```python
from build123d import *
from build123d.topology import SkipClean

# Parameters (mm, degrees)
SWEEP1_PROFILE_R = 12.5


with BuildPart() as part:
    # Sweep1: sweep along a path in Sketch1
    with BuildLine(Plane.XY) as sweep1_path:
        Line((120, -20), (20, -20))
        ThreePointArc((20, -20), (5.857864376, -14.142135624), (0, 0))
        Line((0, 0), (0, 314.65))
        ThreePointArc((0, 314.65), (-8.037977367, 341.838024139), (-29.567546263, 360.28457937))
        Line((-29.567546263, 360.28457937), (-73.011665824, 379.736275328))
    # Sweep1 profile (on start of the path) → Sweep1 (sweep)
    with BuildSketch(Plane(origin=(120, -20, 0), x_dir=(0, 0, -1), z_dir=(-1, 0, 0))):
        Circle(SWEEP1_PROFILE_R)
    sweep(path=sweep1_path.line)

    # Sketch16 → Revolve1 (revolve)
    with SkipClean():  # the faces are left unmerged after this step: merging them gives an invalid solid
        with BuildSketch(Plane.XY):
            with BuildLine():
                Line((120, -7.5), (120, -32.5))
                ThreePointArc((120, -32.5), (132.5, -20), (120, -7.5))
            make_face()
        revolve(axis=Axis((120, -7.5, 0), (0, -1, 0)))


solid = part.part
```
Source: CAD feature listing. Evaluate the final solid. Frame: model axes, mm. Coordinates: 2 decimals unless noted, no trailing zeros. Order: outer loops, then holes, each group sorted by start corner. A loop starts at its lowest first (then second) coordinate and runs counter-clockwise, first axis right, second up. Notation, with made-up numbers: M 35.5,52.5 L 50.5,52.5 A22 ccw 50.5,86.5 Z; hole C 4.25,46 d1. An arc over 180 degrees is marked long. Write each question's results on one line, items separated by ' | '. Start each with the question number.
1) Section query B-B (y = 157). Return the cut outline in (x, z).
2) Contact query for flat-ended pins moving along their axis: pin 1 Ø2 at (x, z) = (0, 4.5) entering from -Y; pin 2 Ø5 at (y, z) = (312.5, 7.5) entering from -X; pin 3 Ø3 at (x, z) = (-18, 2) entering from -Y. Output: stop coordinate, or through.
3) Section query A-A (x = 24). Return the cut outline in (y, z).
4) Draft query along X for faces 1 (the face through (69.3, -8.91, -5.77)), 2 (the face through (-3.755, 159.528, -11.923)), 3 (the face through (-72.94, 379.9, 0.18)). Return one class per face: released by +X, released by -X, zero draft, split by the parting line, or undercut.
5) Line query: line 1 (X direction, y = 223.5, z = 0.5); line 2 (X direction, y = 28.5, z = 1.25); line 3 (Y direction, x = 70, z = 0.75). Output: solid intervals per line, ascending. Write a range as from..to.
Answers:
1) outline: C 0,0 d25
2) pin 1: stops at y = -25.45 | pin 2: stops at x = -11.46 | pin 3: stops at y = 331.82
3) outline: C -20,0 d25
4) face 1: zero draft | face 2: split by the parting line | face 3: released by -X
5) line 1: x = -12.49..12.49 | line 2: x = -12.44..12.44 | line 3: y = -32.48..-7.52
